Source: CAD feature listing. Evaluate the final solid. Frame: model axes, mm. Face numbers are marked on the shaded views. Round coordinates to 2 decimals unless told otherwise and drop trailing zeros. Order: outer loops, then holes, each group sorted by start corner. A loop starts at its lowest first (then second) coordinate and runs counter-clockwise, first axis right, second up. Notation, with made-up numbers: (60, 64.25) - (111, 64.25) arc R25 ccw to (111, 83.25) - close; hole circle Ø6 at (27.5, 25.25). An arc over 180 degrees is marked (long way). Put each result on its own line as item: value. Start each with the question number.
1) Contact query for flat-ended pins moving along their axis: P1, Ø8.5, axis at x = -15.5, y = -15.5, coming from the -Z side; P2, Ø5.5, axis at x = -15.5, y = 15.5, coming from the +Z side. Output: stop coordinate, or through.
2) Section B-B on z = 1.75. Output: boundary loops of the cut face in (x, y).
3) Mould query, pull axis Y, two halves, no side actions, for the marked faces 1, 2 and 3. Classes: +Y half, -Y half, draft (parallel to the pull), parting line (faces both ways), or undercut.
4) Section C-C on y = 15.5. Output: boundary loops of the cut face in (x, z), then the cut area to 3 significant figures.
5) Section A-A on x = 15.5. Output: boundary loops of the cut face in (y, z).
6) Line query: probe 1 along Y at (x, z) = (-15.5, 2.95); probe 2 along Y at (x, z) = (17.5, 0); probe 3 along Y at (x, z) = (0, 2.25). Output: solid intervals per line, ascending. Write a range as [from, to].
```python
from build123d import *

# Parameters (mm, degrees)
SKETCH_1_W                   = 42
SKETCH_1_H                   = 42
EXTRUDE_1_DEPTH              = 4
SKETCH_2_R                   = 11
CUT_EXTRUDE_1_DEPTH          = 31.757112998
HOLE_WIZARD_M3_1_D           = 3.4
HOLE_WIZARD_M3_1_CBORE_D     = 6.5
HOLE_WIZARD_M3_1_CBORE_DEPTH = 3
PATTERN_CIRCULAR_1_COUNT     = 4
M3X0_5_1_D                   = 2.5
M3X0_5_1_DEPTH               = 10
M3X0_5_1_TIP                 = 0.751075774


with BuildPart() as part:
    # 草圖1 → 填料-伸長1 (new, symmetric)
    with BuildSketch(Plane.XY):
        Rectangle(SKETCH_1_W, SKETCH_1_H)
    extrude(amount=EXTRUDE_1_DEPTH, both=True)

    # 草圖2 → 除料-伸長1 (cut, through all)
    with BuildSketch(Plane.XY.offset(4)):
        Circle(SKETCH_2_R)
    extrude(amount=-CUT_EXTRUDE_1_DEPTH, mode=Mode.SUBTRACT)

    # M3 凹頭蓋螺釘的柱孔1 (through all)
    with Locations(Plane.XY.offset(4)):
        with Locations((-15.5, 15.5)):
            hole_wizard_m3_1 = CounterBoreHole(HOLE_WIZARD_M3_1_D / 2, HOLE_WIZARD_M3_1_CBORE_D / 2, HOLE_WIZARD_M3_1_CBORE_DEPTH)

    # 環狀複製排列1: M3 凹頭蓋螺釘的柱孔1 ×4 about axis
    pattern_circular_1_axis = Axis((0, 0, 0), (0, 0, 1))
    for i in range(1, PATTERN_CIRCULAR_1_COUNT):
        add(hole_wizard_m3_1.rotate(pattern_circular_1_axis, i * 360 / PATTERN_CIRCULAR_1_COUNT), mode=Mode.SUBTRACT)

    # M3x0.5 螺紋孔1
    with Locations(Plane(origin=(21, 0, 0), x_dir=(0, 0, -1), z_dir=(1, 0, 0))):
        with Locations((0, 8), (0, -8)):
            Hole(M3X0_5_1_D / 2, depth=M3X0_5_1_DEPTH)
            with Locations((0, 0, -(M3X0_5_1_DEPTH + M3X0_5_1_TIP / 2))):  # 118° drill point
                Cone(0, M3X0_5_1_D / 2, M3X0_5_1_TIP, mode=Mode.SUBTRACT)


solid = part.part
```
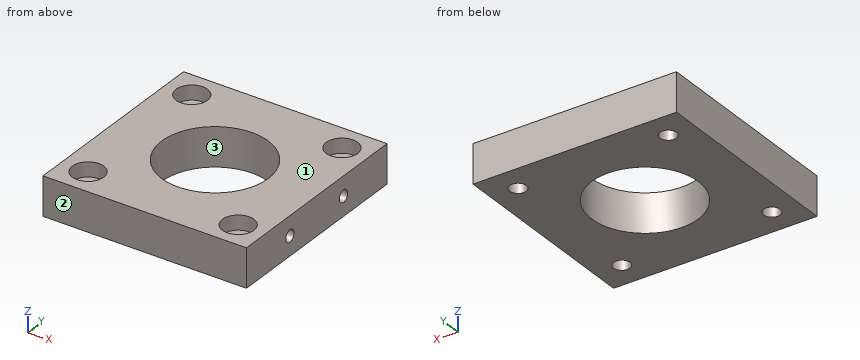
Answer sheet:
1. P1: z = -4
1. P2: z = 1
2. outline: (-21, -21) - (21, -21) - (21, 21) - (-21, 21) - close; hole circle Ø6.5 at (-15.5, -15.5); hole circle Ø6.5 at (-15.5, 15.5); hole circle Ø22 at (0, 0); hole circle Ø6.5 at (15.5, -15.5); hole circle Ø6.5 at (15.5, 15.5)
3. face 1: draft
3. face 2: -Y half
3. face 3: undercut
4. outline: (-21, -4) - (-17.2, -4) - (-17.2, 1) - (-18.75, 1) - (-18.75, 4) - (-21, 4) - close; (-13.8, -4) - (13.8, -4) - (13.8, 1) - (12.25, 1) - (12.25, 4) - (-12.25, 4) - (-12.25, 1) - (-13.8, 1) - close; (17.2, -4) - (21, -4) - (21, 4) - (18.75, 4) - (18.75, 1) - (17.2, 1) - close
4. area: 263 mm^2
5. outline: (-21, -4) - (-17.2, -4) - (-17.2, 1) - (-18.75, 1) - (-18.75, 4) - (-21, 4) - close; (-13.8, -4) - (13.8, -4) - (13.8, 1) - (12.25, 1) - (12.25, 4) - (-12.25, 4) - (-12.25, 1) - (-13.8, 1) - close; (17.2, -4) - (21, -4) - (21, 4) - (18.75, 4) - (18.75, 1) - (17.2, 1) - close; hole circle Ø2.5 at (-8, 0); hole circle Ø2.5 at (8, 0)
6. probe 1: [-21, -18.75], [-12.25, 12.25], [18.75, 21]
6. probe 2: [-21, -9.25], [-6.75, 6.75], [9.25, 21]
6. probe 3: [-21, -11], [11, 21]
